```python
from build123d import *

# Parameters (mm, degrees)
SKETCH1_R           = 0.5
BOSS_EXTRUDE1_DEPTH = 30
SKETCH2_R           = 0.840836639
BOSS_EXTRUDE2_DEPTH = 0.2
DOME1_FACE_RADIUS   = 0.840836639
DOME1_HEIGHT        = 0.5
SCALE1_SCALE        = 1.9329
SCALE2_SCALE        = 1.5


with BuildPart() as part:
    # Sketch1 → Boss-Extrude1 (new body)
    with BuildSketch(Plane.XY):
        Circle(SKETCH1_R)
    extrude(amount=BOSS_EXTRUDE1_DEPTH)

    # Sketch2 → Boss-Extrude2 (add)
    with BuildSketch(Plane(origin=(0, 0, 0), x_dir=(-1, 0, 0), z_dir=(0, 0, -1))):
        Circle(SKETCH2_R)
    extrude(amount=BOSS_EXTRUDE2_DEPTH)

    # Dome1: a dome of height H over a round flat face of radius A is a cap of a sphere of radius (A * A + H * H) / (2 * H)
    dome1_r = (DOME1_FACE_RADIUS * DOME1_FACE_RADIUS + DOME1_HEIGHT * DOME1_HEIGHT) / (2 * DOME1_HEIGHT)
    dome1_base = Plane((0, 0, -0.2), z_dir=(0, 0, -1))
    with Locations(dome1_base.offset(DOME1_HEIGHT - dome1_r)):
        dome1_ball = Sphere(dome1_r, mode=Mode.PRIVATE)
    add(split(dome1_ball, bisect_by=dome1_base, keep=Keep.TOP, mode=Mode.PRIVATE))


with BuildPart() as part_1:
    # Scale1: scaled about (0, 0, 14.340078406)
    add(part.part.scale(SCALE1_SCALE).moved(Location((0, 0, -13.377859145))))


with BuildPart() as part_2:
    # Scale2: scaled about (0, 0, 14.340078406)
    add(part_1.part.scale(SCALE2_SCALE).moved(Location((0, 0, -7.170039203))))


solid = part_2.part
```
Here's how the part is built. I have some questions about the finished solid (model axes, mm). A direction names the side the tool comes from. Coordinates: 2 decimals unless noted, no trailing zeros. Order: outer loops, then holes, each group sorted by start corner. A loop starts at its lowest first (then second) coordinate and runs counter-clockwise, first axis right, second up.
Item 1: If we section it at C-C, the plane z = -0.5: List the corners of the cut face in (x, y) for me, then the cut area to 3 significant figures.
Response values:
outline: circle Ø2.9 at (0, 0)
area: 6.60 mm2
Item 2: I need wall thicknesses on probe 1 along Y at (x, z) = (-0.1, 6); probe 2 along Z at (x, y) = (0.3, 0.05); probe 3 along X at (y, z) = (-0.7, -17). Which ranges of each line are inside material? Lowest first, please.
Response values:
probe 1: y = -1.45 to 1.45
probe 2: z = -29.25 to 59.74
probe 3: x = -1.27 to 1.27
Item 3: Which directions (+Z, -Z, +X, -X, +Y, -Y) give clear straight access to the entire face, cutting with the end or side of a thin tool? Please do faces 1 (the face through (1.935, -1.483, -27.523)), 2 (the face through (0, -2, -27.237)).
Response values:
face 1: +Z, -Z
face 2: +Z
Item 4: If we section it at A-A, the plane y = 0: List the corners of the cut face in (x, z) for me.
Response values:
outline: (-2.44, -27.82) arc R2.77 ccw to (2.44, -27.82) - (2.44, -27.24) - (1.45, -27.24) - (1.45, 59.74) - (-1.45, 59.74) - (-1.45, -27.24) - (-2.44, -27.24) - close
Item 5: I'm going to push flat-ended pins straight in: pin 1 Ø2 at (x, z) = (-0.5, 43) entering from +Y; pin 2 Ø1 at (x, y) = (-1, 0) entering from -Z; pin 3 Ø1.5 at (x, z) = (0.5, 18) entering from -Y. Where does each tip first touch, or does it pass through?
Response values:
pin 1: stops at y = 1.45
pin 2: stops at z = -29.22
pin 3: stops at y = -1.45
